Could you check a few things on this model? Use its own coordinates, in mm. Face numbers are marked on the shaded views. A direction names the side the tool comes from. Give positions to 0.01 mm unless a question says otherwise; leave off trailing zeros. Write each loop counter-clockwise with the first axis right and the second up, starting at its lowest first coordinate (ties: lowest second). Pieces come first, ordered by that corner, then holes. Notation, with made-up numbers: M -38,43.25 L -12,43.25 A30 ccw -12,81.25 Z; hole C -28.5,-3 d8. An arc over 180 degrees is marked long. Answer as CSV lines item,"result". Start each with the question number.
from build123d import *

# Parameters (mm, degrees)
BOSS_EXTRU_1_DEPTH      = 672
ENL_V_MAT_EXTRU_1_DEPTH = 590
ENL_V_MAT_EXTRU_2_DEPTH = 590


with BuildPart() as part:
    # Esquisse1 → Boss.-Extru.1 (new body)
    with BuildSketch(Plane(origin=(0, 0, 0), x_dir=(1, 0, 0), z_dir=(0, 1, 0))):
        Polygon((-20, 20.113636364), (20, 20.113636364), (20, 18.113636364), (-18, 18.113636364), (-18, -19.886363636), (-20, -19.886363636), align=None)
    extrude(amount=BOSS_EXTRU_1_DEPTH)

    # Esquisse2 → Enlèv. mat.-Extru.1 (cut)
    with BuildSketch(Plane(origin=(0, 0, -20.113636364), x_dir=(-1, 0, 0), z_dir=(0, 0, -1))):
        Polygon((20, 0), (-20, 40), (-20, 0), align=None)
    extrude(amount=-ENL_V_MAT_EXTRU_1_DEPTH, mode=Mode.SUBTRACT)

    # Esquisse3 → Enlèv. mat.-Extru.2 (cut)
    with BuildSketch(Plane.ZY.offset(20)):
        Polygon((-20.113636364, 0), (19.886363636, 40), (19.886363636, 0), align=None)
    extrude(amount=-ENL_V_MAT_EXTRU_2_DEPTH, mode=Mode.SUBTRACT)


solid = part.part
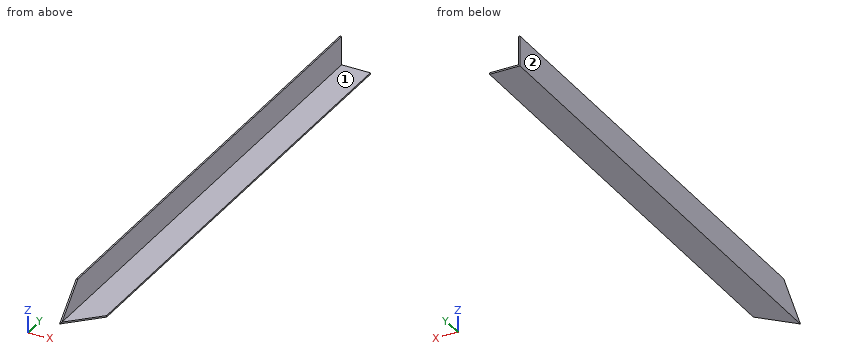
1. Imagine slicing it at C-C, the plane z = 1. Please give me the cut outline in (x, y).
2. Imagine slicing it at A-A, the plane y = 56. Please give me the cut outline in (x, z).
3. Imagine slicing it at B-B, the plane x = 10. Please give me the cut outline in (y, z), plus the area to 3 significant figures.
4. On a 3-axis mill with a long thin cutter (end or side, diameter ignored), from which of +Z, -Z, +X, -X, +Y, -Y can I reach the whole of each face in a straight line? I mean the marked faces 1 and 2. Say none if no direction works.
5. Please list where these lines run through material, in increasing order: line 1 (X direction, y = 552, z = 0); line 2 (Z direction, x = -7, y = 270).
6. Will this pin go through, and if not, where does the flat tip stop? P1, Ø3, axis at y = 596, z = -14.5, coming from the +X side.
Solutions:
1,outline,"M -20,21.11 L -18,21.11 L -18,672 L -20,672 Z"
2,outline,"M -20,-20.11 L 20,-20.11 L 20,-18.11 L -18,-18.11 L -18,19.89 L -20,19.89 Z"
3,outline,"M 30,-20.11 L 672,-20.11 L 672,-18.11 L 30,-18.11 Z"
3,area,"1,280 mm²"
4,face 1,"+Z, +X, +Y, -Y"
4,face 2,"+Z, -Z, -X, +Y, -Y"
5,line 1,"-20 to -18"
5,line 2,"-20.11 to -18.11"
6,P1,"x = -18"
